```python
from build123d import *

# Parameters (mm, degrees)
BOSS_EXTRUDE1_DEPTH = 12


with BuildPart() as part:
    # Sketch1 → Boss-Extrude1 (new body)
    with BuildSketch(Plane.XY):
        with BuildLine():
            Line((-298.012610176, -63.342318059), (45.11407446, -63.342318059))
            ThreePointArc((45.11407446, -63.342318059), (87.540481331, -80.915911188), (105.11407446, -123.342318059))
            Line((105.11407446, -123.342318059), (105.11407446, -168.342318059))
            ThreePointArc((105.11407446, -168.342318059), (118.294269306, -200.162123213), (150.11407446, -213.342318059))
            Line((150.11407446, -213.342318059), (277.389007074, -213.342318059))
            Line((277.389007074, -213.342318059), (281.987389824, -213.342318059))
            ThreePointArc((281.987389824, -213.342318059), (296.129525447, -207.484453683), (301.987389824, -193.342318059))
            Line((301.987389824, -193.342318059), (301.987389824, -63.342318059))
            Line((301.987389824, -63.342318059), (301.987389824, -16.342318059))
            Line((301.987389824, -16.342318059), (293.265850793, -16.342318059))
            ThreePointArc((293.265850793, -16.342318059), (289.490333549, -16.839374334), (289.987389824, -13.06385709))
            Line((289.987389824, -13.06385709), (289.987389824, 27.379220972))
            ThreePointArc((289.987389824, 27.379220972), (289.490333549, 31.154738216), (293.265850793, 30.657681941))
            Line((293.265850793, 30.657681941), (301.987389824, 30.657681941))
            Line((301.987389824, 30.657681941), (301.987389824, 77.657681941))
            Line((301.987389824, 77.657681941), (293.265850793, 77.657681941))
            ThreePointArc((293.265850793, 77.657681941), (289.490333549, 77.160625666), (289.987389824, 80.93614291))
            Line((289.987389824, 80.93614291), (289.987389824, 124.657681941))
            Line((289.987389824, 124.657681941), (255.265850793, 124.657681941))
            ThreePointArc((255.265850793, 124.657681941), (251.490333549, 124.160625666), (251.987389824, 127.93614291))
            Line((251.987389824, 127.93614291), (251.987389824, 136.657681941))
            Line((251.987389824, 136.657681941), (201.987389824, 136.657681941))
            Line((201.987389824, 136.657681941), (201.987389824, 127.93614291))
            ThreePointArc((201.987389824, 127.93614291), (202.484446099, 124.160625666), (198.708928855, 124.657681941))
            Line((198.708928855, 124.657681941), (155.265850793, 124.657681941))
            ThreePointArc((155.265850793, 124.657681941), (151.490333549, 124.160625666), (151.987389824, 127.93614291))
            Line((151.987389824, 127.93614291), (151.987389824, 136.657681941))
            Line((151.987389824, 136.657681941), (101.987389824, 136.657681941))
            Line((101.987389824, 136.657681941), (101.987389824, 127.93614291))
            ThreePointArc((101.987389824, 127.93614291), (102.484446099, 124.160625666), (98.708928855, 124.657681941))
            Line((98.708928855, 124.657681941), (-94.734149207, 124.657681941))
            ThreePointArc((-94.734149207, 124.657681941), (-98.509666451, 124.160625666), (-98.012610176, 127.93614291))
            Line((-98.012610176, 127.93614291), (-98.012610176, 136.657681941))
            Line((-98.012610176, 136.657681941), (-148.012610176, 136.657681941))
            Line((-148.012610176, 136.657681941), (-148.012610176, 127.93614291))
            ThreePointArc((-148.012610176, 127.93614291), (-147.515553901, 124.160625666), (-151.291071145, 124.657681941))
            Line((-151.291071145, 124.657681941), (-194.734149207, 124.657681941))
            ThreePointArc((-194.734149207, 124.657681941), (-198.509666451, 124.160625666), (-198.012610176, 127.93614291))
            Line((-198.012610176, 127.93614291), (-198.012610176, 136.657681941))
            Line((-198.012610176, 136.657681941), (-248.012610176, 136.657681941))
            Line((-248.012610176, 136.657681941), (-248.012610176, 127.93614291))
            ThreePointArc((-248.012610176, 127.93614291), (-247.515553901, 124.160625666), (-251.291071145, 124.657681941))
            Line((-251.291071145, 124.657681941), (-286.012610176, 124.657681941))
            Line((-286.012610176, 124.657681941), (-286.012610176, 80.93614291))
            ThreePointArc((-286.012610176, 80.93614291), (-285.515553901, 77.160625666), (-289.291071145, 77.657681941))
            Line((-289.291071145, 77.657681941), (-298.012610176, 77.657681941))
            Line((-298.012610176, 77.657681941), (-298.012610176, 30.657681941))
            Line((-298.012610176, 30.657681941), (-289.291071145, 30.657681941))
            ThreePointArc((-289.291071145, 30.657681941), (-285.515553901, 31.154738216), (-286.012610176, 27.379220972))
            Line((-286.012610176, 27.379220972), (-286.012610176, -13.06385709))
            ThreePointArc((-286.012610176, -13.06385709), (-285.515553901, -16.839374334), (-289.291071145, -16.342318059))
            Line((-289.291071145, -16.342318059), (-298.012610176, -16.342318059))
            Line((-298.012610176, -16.342318059), (-298.012610176, -63.342318059))
        make_face()
    extrude(amount=BOSS_EXTRUDE1_DEPTH)


solid = part.part
```
Model file for the job. Use its own axes, mm. A direction names the side the tool comes from. Give positions to 0.01 mm unless a question says otherwise; leave off trailing zeros. Loops run counter-clockwise (first coordinate to the right, second up) from the corner with the lowest first, then second, coordinate; pieces in that order, holes last. Notation, with made-up numbers: (49.25, 10) - (71.25, 10) arc R4 ccw to (71.25, 17) - close; hole circle Ø10 at (53, -22.75). An arc over 180 degrees is marked (long way). One line per item, written item: value. Start each with the question number.
1. Slice it at A-A (y = 89.5). List the corners of the cut face in (x, z).
2. Probe L1, parallel to Y at x = 271.5, z = 9.25; L2, parallel to X at y = 8.5, z = 0.5; L3, parallel to X at y = -135, z = 9. List the from-to ranges inside material, lowest first. Write a range as from..to.
3. Which spindle directions (+Z, -Z, +X, -X, +Y, -Y) get a long thin tool onto all of the face, cutting with end or side? Do faces 1 (the flat face through (273, 124.658, 6)), 2 (the flat face through (289.987, 7, 6)), 3 (the flat face through (-173, 124.658, 6)), 4 (the flat face through (-286.013, 103, 6)), 5 (the flat face through (-129, -63.342, 6)). Say none if no direction does.
4. Slice it at B-B (x = -177). List the corners of the cut face in (y, z), plus the area to 3 significant figures.
5. Pin check, flat tips, straight feed: pin 1 (4.5 mm diameter, centred on x = -292, z = 5, fed in from +Y); pin 2 (3.5 mm diameter, centred on y = 105, z = 6, fed in from -X); pin 3 (6 mm diameter, centred on y = -136, z = 3.5, fed in from -X). Stop position of each tip, or through.
6. Pull direction X, two halves, no side cores. Call faces 6 (the cylindrical face through (117.946, -199.81, 5.916)), 7 (the flat face through (-223, 136.658, 6)), 8 (the flat face through (177, 124.658, 6)): pulls with the +X half, pulls with the -X half, needs draft (parallel to the pull), parting line crosses it, or undercut.
Solution:
1. outline: (-286.01, 0) - (289.99, 0) - (289.99, 12) - (-286.01, 12) - close
2. L1: y = -213.34..124.66
2. L2: x = -286.01..289.99
2. L3: x = 105.11..301.99
3. face 1: +Z, -Z, +X, +Y
3. face 2: +Z, -Z, +X
3. face 3: +Z, -Z, +Y
3. face 4: +Z, -Z, -X, +Y
3. face 5: +Z, -Z, -X, -Y
4. outline: (-63.34, 0) - (124.66, 0) - (124.66, 12) - (-63.34, 12) - close
4. area: 2,260 mm^2
5. pin 1: stops at y = 77.66
5. pin 2: stops at x = -286.01
5. pin 3: stops at x = 105.11
6. face 6: pulls with the -X half
6. face 7: needs draft
6. face 8: undercut
